Work out the finished part from the listing and answer in its coordinate system (mm). A direction names the side the tool comes from. Coordinates: 2 decimals unless noted, no trailing zeros. Write each loop counter-clockwise with the first axis right and the second up, starting at its lowest first coordinate (ties: lowest second). Pieces come first, ordered by that corner, then holes. Notation, with made-up numbers: (-21.75, 83) - (-15.75, 83) arc R35 ccw to (-15.75, 115) - close; hole circle Ø6 at (57, 45.5). An arc over 180 degrees is marked (long way). Use CSV: the item, a comma, the result in double quotes. Start each with the question number.
from build123d import *

# Parameters (mm, degrees)
ESBO_O1_W                = 30
ESBO_O1_H                = 20
RESSALTO_EXTRUS_O1_DEPTH = 3
ESBO_O2_R                = 8.2
CORTE_EXTRUS_O1_DEPTH    = 20
FILETE1_R                = 10
ESBO_O3_W                = 8
ESBO_O3_H                = 6
RESSALTO_EXTRUS_O2_DEPTH = 2
ESBO_O4_W                = 12
ESBO_O4_H                = 6
RESSALTO_EXTRUS_O3_DEPTH = 2
CHANFRO1_SIZE            = 2


with BuildPart() as part:
    # Esboço1 → Ressalto-extrusão1 (new, symmetric)
    with BuildSketch(Plane(origin=(0, 0, 0), x_dir=(1, 0, 0), z_dir=(0, 1, 0))):
        Rectangle(ESBO_O1_W, ESBO_O1_H)
    extrude(amount=RESSALTO_EXTRUS_O1_DEPTH, both=True)

    # Esboço2 → Corte-extrusão1 (cut, through all)
    with BuildSketch(Plane(origin=(0, 3, 0), x_dir=(1, 0, 0), z_dir=(0, 1, 0))):
        with Locations(Location((5, 0, 0), (0, 0, 270))):
            Circle(ESBO_O2_R)
    extrude(amount=-CORTE_EXTRUS_O1_DEPTH, mode=Mode.SUBTRACT)

    # Filete1
    filete1_edges = [part.edges().sort_by_distance(p)[0] for p in [
        (15, 0, -10),
        (15, 0, 10),
    ]]
    fillet(filete1_edges, radius=FILETE1_R - 0.0001)  # a hair under: the kernel refuses the full size

    # Esboço3 → Ressalto-extrusão2 (add)
    with BuildSketch(Plane.ZY.offset(15)):
        Rectangle(ESBO_O3_W, ESBO_O3_H)
    extrude(amount=RESSALTO_EXTRUS_O2_DEPTH)

    # Esboço4 → Ressalto-extrusão3 (add)
    with BuildSketch(Plane.ZY.offset(17)):
        Rectangle(ESBO_O4_W, ESBO_O4_H)
    extrude(amount=RESSALTO_EXTRUS_O3_DEPTH)

    # Chanfro1
    chanfro1_edges = [part.edges().sort_by_distance(p)[0] for p in [
        (-19, 0, 6),
        (-19, 0, -6),
    ]]
    chamfer(chanfro1_edges, length=CHANFRO1_SIZE - 0.0001)  # a hair under: the kernel refuses the full size


solid = part.part
Item 1: Straight lines are drawn through the part: probe 1 along X at (y, z) = (0.75, 0); probe 2 along X at (y, z) = (-1.75, -1); probe 3 along Z at (x, y) = (11.5, -1.5). For each, find the intervals that lie inside material, in ascending order. Write a range as [from, to].
Item 2: Which of the six approach directions +Z, -Z, +X, -X, +Y, -Y give full straight-line access (tool end or side, diameter ignored) to faces 1 (the face through (11.99, -0.04, -7.15)), 2 (the face through (-16, 0, 4)), 3 (the face through (-15, 0, -7))?
Item 3: A cutting plane is placed at C-C (x = 1.5). Determine the outline of the cut face in (y, z), then the cut area to 3 significant figures.
Item 4: Determine the mould class of faces 4 (the face through (-17, 0, -5)), 5 (the face through (-18, 0, 5)), 6 (the face through (7.463, 0.042, 7.821)) for opening direction Z: +Z half, -Z half, draft (parallel to the pull), parting line (faces both ways), or undercut.
Item 5: Each of these flat-tipped pins is pushed along its axis until it touches: pin 1 (1.5 mm diameter, centred on y = 2, z = -5, fed in from +X); pin 2 (1 mm diameter, centred on y = -1, z = 4.5, fed in from +X); pin 3 (1.6 mm diameter, centred on x = -16.5, y = -1, fed in from +Z). Where does it stop, or does it pass through?
Item 6: A cutting plane is placed at B-B (z = 1.75). Determine the outline of the cut face in (x, y), then the cut area to 3 significant figures.
Calculated:
1,probe 1,"x = [-19, -3.2], [13.2, 15]"
1,probe 2,"x = [-19, -3.14], [13.14, 14.95]"
1,probe 3,"z = [-7.6, -5], [5, 7.6]"
2,face 1,"-Z, +X, +Y, -Y"
2,face 2,"+Z, +Y, -Y"
2,face 3,"-Z, +Y, -Y"
3,outline,"(-3, -10) - (3, -10) - (3, -7.42) - (-3, -7.42) - close; (-3, 7.42) - (3, 7.42) - (3, 10) - (-3, 10) - close"
3,area,"31.0 mm²"
4,face 4,"draft"
4,face 5,"+Z half"
4,face 6,"undercut"
5,pin 1,"stops at x = 14.05"
5,pin 2,"stops at x = 14.17"
5,pin 3,"stops at z = 6"
6,outline,"(-19, -3) - (-3.01, -3) - (-3.01, 3) - (-19, 3) - close; (13.01, -3) - (14.85, -3) - (14.85, 3) - (13.01, 3) - close"
6,area,"107 mm²"
